```python
from build123d import *

# Parameters (mm, degrees)
BOSS_EXTRUDE1_DEPTH = 17.5
SKETCH2_W           = 20
SKETCH2_H           = 20
CUT_EXTRUDE1_DEPTH  = 64.492125496
SKETCH3_R           = 2
CUT_EXTRUDE2_DEPTH  = 71.356236397
CHAMFER1_SIZE       = 3
CHAMFER2_SIZE       = 5
FILLET1_RADIUS      = 6
FILLET1_LENGTH      = 5
SKETCH4_R           = 2.5
CUT_EXTRUDE3_DEPTH  = 35
FILLET2_R           = 5
FILLET3_R           = 1


with BuildPart() as part:
    # Sketch1 → Boss-Extrude1 (new, symmetric)
    with BuildSketch(Plane(origin=(0, 0, 0), x_dir=(0, 0, -1), z_dir=(1, 0, 0))):
        Polygon((0, 0), (-35, 0), (-35, -20), (-12, -20), (-12, -50), (0, -50), align=None)
    extrude(amount=BOSS_EXTRUDE1_DEPTH, both=True)

    # Sketch2 → Cut-Extrude1 (cut, through all)
    with BuildSketch(Plane(origin=(0, 0, 0), x_dir=(-1, 0, 0), z_dir=(0, 0, -1))):
        Polygon((17.5, -25), (2.5, -30.459553514), (2.5, -50), (17.5, -50), align=None)
        Polygon((-17.5, -50), (-17.5, -25), (-2.5, -30.459553514), (-2.5, -50), align=None)
        with Locations((0, -10)):
            Rectangle(SKETCH2_W, SKETCH2_H)
    extrude(amount=-CUT_EXTRUDE1_DEPTH, mode=Mode.SUBTRACT)

    # Sketch3 → Cut-Extrude2 (cut, through all)
    with BuildSketch(Plane.ZY.offset(17.5)):
        with Locations((5, -8)):
            Circle(SKETCH3_R)
        with Locations((30, -8)):
            Circle(SKETCH3_R)
    extrude(amount=-CUT_EXTRUDE2_DEPTH, mode=Mode.SUBTRACT)

    # Chamfer1
    chamfer1_edges = [part.edges().sort_by_distance(p)[0] for p in [
        (13.75, -20, 12),
        (13.75, -20, 35),
        (13.75, 0, 35),
        (13.75, 0, 0),
        (-13.75, -20, 12),
        (-13.75, -20, 35),
        (-13.75, 0, 35),
        (-13.75, 0, 0),
    ]]
    chamfer(chamfer1_edges, length=CHAMFER1_SIZE)

    # Chamfer2
    chamfer2_edges = [part.edges().sort_by_distance(p)[0] for p in [
        (-10, -20, 6),
        (10, -20, 6),
    ]]
    chamfer(chamfer2_edges, length=CHAMFER2_SIZE)

    # Fillet1: full round fillet: the end face becomes a half cylinder, R = half its width
    fillet1_face = Plane((0, -50, 6), x_dir=(1, 0, 0), z_dir=(0, -1, 0))  # on the end face: x along it, z out of the body
    fillet1_slab = fillet1_face.offset(-FILLET1_RADIUS / 2) * Box(FILLET1_LENGTH, 2 * FILLET1_RADIUS, FILLET1_RADIUS, mode=Mode.PRIVATE)  # the body's end, R deep
    fillet1_round = Plane((0, -44, 6), x_dir=(0, -1, 0), z_dir=(1, 0, 0)) * Cylinder(FILLET1_RADIUS, FILLET1_LENGTH, mode=Mode.PRIVATE)  # its axis R under the face
    add(fillet1_slab - fillet1_round, mode=Mode.SUBTRACT)

    # Sketch4 → Cut-Extrude3 (cut)
    with BuildSketch(Plane(origin=(2.5, 0, 0), x_dir=(0, 0, -1), z_dir=(1, 0, 0))):
        with Locations(Location((-6, -44, 0), (0, 0, 90))):
            Circle(SKETCH4_R)
    extrude(amount=-CUT_EXTRUDE3_DEPTH, mode=Mode.SUBTRACT)

    # Fillet2
    # the kernel refuses this fillet: 5 mm, written as the material it adds along each edge
    with BuildSketch(Plane(origin=(10, -35.5, 12), x_dir=(-1, 0, 0), z_dir=(0, 1, 0))) as fillet2_piece_1_section:
        with BuildLine():
            CenterArc((FILLET2_R, FILLET2_R), FILLET2_R, 180, 90)
            Line((0, FILLET2_R), (0, 0))
            Line((0, 0), (FILLET2_R, 0))
        make_face()
    fillet2_piece_1 = extrude(amount=33, mode=Mode.PRIVATE)
    fillet2_piece_1 = split(fillet2_piece_1, bisect_by=Plane(origin=(9.996559124, -19.16276417, 15.83723583), z_dir=(0, -0.7071067811865476, 0.7071067811865476)), keep=Keep.TOP, mode=Mode.PRIVATE)
    fillet2_piece_1 = split(fillet2_piece_1, bisect_by=Plane(origin=(9.996559124, -20, 16.11631444), z_dir=(0, 1, 0)), keep=Keep.TOP, mode=Mode.PRIVATE)
    add(fillet2_piece_1)
    with BuildSketch(Plane(origin=(10, -35.5, 12), x_dir=(-1, 0, 0), z_dir=(0, 1, 0))) as fillet2_piece_2_section:
        with BuildLine():
            CenterArc((FILLET2_R, FILLET2_R), FILLET2_R, 180, 90)
            Line((0, FILLET2_R), (0, 0))
            Line((0, 0), (FILLET2_R, 0))
        make_face()
    fillet2_piece_2 = extrude(amount=33, mode=Mode.PRIVATE)
    fillet2_piece_2 = split(fillet2_piece_2, bisect_by=Plane(origin=(8.541566655, -21.793394373, 13.206605627), z_dir=(0, 0.7071067811865476, -0.7071067811865476)), keep=Keep.TOP, mode=Mode.PRIVATE)
    fillet2_piece_2 = split(fillet2_piece_2, bisect_by=Plane(origin=(8.541566655, -20, 12.608807503), z_dir=(0, -1, 0)), keep=Keep.TOP, mode=Mode.PRIVATE)
    add(fillet2_piece_2)
    with BuildSketch(Plane(origin=(10, -35.5, 12), x_dir=(-1, 0, 0), z_dir=(0, 1, 0))) as fillet2_piece_3_section:
        with BuildLine():
            CenterArc((FILLET2_R, FILLET2_R), FILLET2_R, 180, 90)
            Line((0, FILLET2_R), (0, 0))
            Line((0, 0), (FILLET2_R, 0))
        make_face()
    fillet2_piece_3 = extrude(amount=33, mode=Mode.PRIVATE)
    fillet2_piece_3 = split(fillet2_piece_3, bisect_by=Plane(origin=(8.131124987, -16.868875013, 13.270711332), z_dir=(0.7071067811865476, -0.7071067811865476, 0)), keep=Keep.TOP, mode=Mode.PRIVATE)
    fillet2_piece_3 = split(fillet2_piece_3, bisect_by=Plane(origin=(9.156989341, -19.812014017, 15.187985983), z_dir=(0, 0.7071067811865476, -0.7071067811865476)), keep=Keep.TOP, mode=Mode.PRIVATE)
    fillet2_piece_3 = split(fillet2_piece_3, bisect_by=Plane(origin=(9.156989341, -20, 13.270711332), z_dir=(0, 1, 0)), keep=Keep.TOP, mode=Mode.PRIVATE)
    add(fillet2_piece_3)
    with BuildSketch(Plane(origin=(-10, -35.5, 12), x_dir=(0, 0, 1), z_dir=(0, 1, 0))) as fillet2_piece_4_section:
        with BuildLine():
            CenterArc((FILLET2_R, FILLET2_R), FILLET2_R, 180, 90)
            Line((0, FILLET2_R), (0, 0))
            Line((0, 0), (FILLET2_R, 0))
        make_face()
    fillet2_piece_4 = extrude(amount=33, mode=Mode.PRIVATE)
    fillet2_piece_4 = split(fillet2_piece_4, bisect_by=Plane(origin=(-8.541566654, -21.793394373, 13.206605627), z_dir=(0, 0.7071067811865476, -0.7071067811865476)), keep=Keep.TOP, mode=Mode.PRIVATE)
    fillet2_piece_4 = split(fillet2_piece_4, bisect_by=Plane(origin=(-8.541566654, -20, 12.608807503), z_dir=(0, -1, 0)), keep=Keep.TOP, mode=Mode.PRIVATE)
    add(fillet2_piece_4)
    with BuildSketch(Plane(origin=(-10, -35.5, 12), x_dir=(0, 0, 1), z_dir=(0, 1, 0))) as fillet2_piece_5_section:
        with BuildLine():
            CenterArc((FILLET2_R, FILLET2_R), FILLET2_R, 180, 90)
            Line((0, FILLET2_R), (0, 0))
            Line((0, 0), (FILLET2_R, 0))
        make_face()
    fillet2_piece_5 = extrude(amount=33, mode=Mode.PRIVATE)
    fillet2_piece_5 = split(fillet2_piece_5, bisect_by=Plane(origin=(-9.996559123, -19.16276417, 15.83723583), z_dir=(0, -0.7071067811865476, 0.7071067811865476)), keep=Keep.TOP, mode=Mode.PRIVATE)
    fillet2_piece_5 = split(fillet2_piece_5, bisect_by=Plane(origin=(-9.996559123, -20, 16.11631444), z_dir=(0, 1, 0)), keep=Keep.TOP, mode=Mode.PRIVATE)
    add(fillet2_piece_5)
    with BuildSketch(Plane(origin=(-10, -35.5, 12), x_dir=(0, 0, 1), z_dir=(0, 1, 0))) as fillet2_piece_6_section:
        with BuildLine():
            CenterArc((FILLET2_R, FILLET2_R), FILLET2_R, 180, 90)
            Line((0, FILLET2_R), (0, 0))
            Line((0, 0), (FILLET2_R, 0))
        make_face()
    fillet2_piece_6 = extrude(amount=33, mode=Mode.PRIVATE)
    fillet2_piece_6 = split(fillet2_piece_6, bisect_by=Plane(origin=(-9.156989342, -19.812014017, 15.187985983), z_dir=(0, 0.7071067811865476, -0.7071067811865476)), keep=Keep.TOP, mode=Mode.PRIVATE)
    fillet2_piece_6 = split(fillet2_piece_6, bisect_by=Plane(origin=(-8.131124988, -16.868875012, 13.270711332), z_dir=(-0.7071067811865476, -0.7071067811865476, 0)), keep=Keep.TOP, mode=Mode.PRIVATE)
    fillet2_piece_6 = split(fillet2_piece_6, bisect_by=Plane(origin=(-9.156989342, -20, 13.270711332), z_dir=(0, 1, 0)), keep=Keep.TOP, mode=Mode.PRIVATE)
    add(fillet2_piece_6)
    with BuildSketch(Plane(origin=(2.5, -30.459553514, 0), x_dir=(0, -1, 0), z_dir=(0, 0, 1)), Plane(origin=(-2.5, -30.459553514, 0), x_dir=(-0.9396926207859091, 0.34202014332566677, 0), z_dir=(0, 0, 1))) as fillet2_piece_7:
        with BuildLine():
            CenterArc((FILLET2_R * 0.70020753821, FILLET2_R), FILLET2_R, 200, 70)
            Line((-FILLET2_R * 0.239485082576, FILLET2_R * 0.657979856674), (0, 0))
            Line((0, 0), (FILLET2_R * 0.70020753821, 0))
        make_face()
    extrude(amount=12)
    # the kernel refuses this fillet: 5 mm, written as the material it takes off along each edge
    with BuildSketch(Plane(origin=(17.5, -25, -8.752594228), x_dir=(0, 1, 0), z_dir=(0, 0, 1))) as fillet2_2_piece_1:
        with BuildLine():
            CenterArc((FILLET2_R * 0.70020753821, FILLET2_R), FILLET2_R, 200, 70)
            Line((-FILLET2_R * 0.239485082576, FILLET2_R * 0.657979856674), (0, 0))
            Line((0, 0), (FILLET2_R * 0.70020753821, 0))
        make_face()
    extrude(amount=29.505188455, mode=Mode.SUBTRACT)
    with BuildSketch(Plane(origin=(-17.5, -25, -8.752594228), x_dir=(0, 1, 0), z_dir=(0, 0, 1))) as fillet2_2_piece_2:
        with BuildLine():
            CenterArc((FILLET2_R * 0.70020753821, -FILLET2_R), FILLET2_R, 90, 70)
            Line((-FILLET2_R * 0.239485082576, -FILLET2_R * 0.657979856674), (0, 0))
            Line((0, 0), (FILLET2_R * 0.70020753821, 0))
        make_face()
    extrude(amount=29.505188455, mode=Mode.SUBTRACT)

    # Fillet3
    fillet3_edges = [part.edges().sort_by_distance(p)[0] for p in [
        (11.134684772, -23, 12),
        (13.541287847, -20, 15),
        (13.75, -20, 32),
        (13.75, -17, 35),
        (13.75, 0, 32),
        (13.75, 0, 3),
        (13.75, -3, 0),
        (13.75, -3, 35),
        (-13.75, -20, 32),
        (-13.541287847, -20, 15),
        (-11.134684772, -23, 12),
        (-13.75, -3, 0),
        (-13.75, 0, 3),
        (-13.75, 0, 32),
        (-13.75, -3, 35),
        (-13.75, -17, 35),
    ]]
    fillet(fillet3_edges, radius=FILLET3_R)


solid = part.part
```
Could you check a few things on this model? Use its own coordinates, in mm. A direction names the side the tool comes from. Round coordinates to 2 decimals unless told otherwise and drop trailing zeros. Loops run counter-clockwise (first coordinate to the right, second up) from the corner with the lowest first, then second, coordinate; pieces in that order, holes last. Notation, with made-up numbers: M -1.5,31 L 8.5,31 A4 cw 8.5,35 Z; hole C -24,-9 d3. An arc over 180 degrees is marked long. Write item = value, one per line.
1. I need wall thicknesses on probe 1 along X at (y, z) = (-13, 28); probe 2 along X at (y, z) = (-37, 5); probe 3 along Y at (x, z) = (15, 30). Which ranges of each line are inside material? Lowest first, please.
Results below:
probe_1 = -17.5 to -10, 10 to 17.5
probe_2 = -2.5 to 2.5
probe_3 = -20 to -10, -6 to 0
2. I want a section at C-C, the plane x = -15. Write out the boundary of the cut face in (y, z).
Results below:
outline = M -25.83,0 L -3.41,0 A1 ccw -2.71,0.29 L -0.29,2.71 A1 ccw 0,3.41 L 0,31.59 A1 ccw -0.29,32.29 L -2.71,34.71 A1 ccw -3.41,35 L -16.59,35 A1 ccw -17.29,34.71 L -19.71,32.29 A1 ccw -20,31.59 L -20,15.41 A1 cw -20.29,14.71 L -22.71,12.29 A1 cw -23.41,12 L -25.83,12 Z; hole C -8,5 d4; hole C -8,30 d4
3. Thinking about a two-plate mould opening in Z: for faces 6 (the face through (13.697, -7.399, 31.908)), 7 (the face through (14, -1, 2)), 8 (the face through (-14, -2, 34)), which applies, +Z half, -Z half, draft (parallel to the pull), parting line (faces both ways), or undercut?
Results below:
face_6 = undercut
face_7 = -Z half
face_8 = +Z half
4. Will these pins go through, and if not, where does the flat tip stop? P1, Ø2.5, axis at x = -14, z = 24, coming from the -Y side; P2, Ø5, axis at x = 0, z = 4.5, coming from the +Y side; P3, Ø13, axis at y = -42, z = 9, coming from the -X side.
Results below:
P1 = -20
P2 = -20
P3 = -2.5
5. Which directions (+Z, -Z, +X, -X, +Y, -Y) give clear straight access to the entire face, cutting with the end or side of a thin tool? Please do faces 1 (the face through (8, -17, 6)), 2 (the face through (14, -20, 23)), 3 (the face through (9, -19, 14)), 4 (the face through (0, -29, 12)), 5 (the face through (2.5, -40, 6)).
Results below:
face_1 = +Z, -Z, +Y
face_2 = +Z, +X, -X, -Y
face_3 = +Z, +Y, -Y
face_4 = +Z, -Y
face_5 = +Z, -Z, +X, -Y
6. I want a section at A-A, the plane z = 30. Write out the boundary of the cut face in (x, y).
Results below:
outline = M -17.5,-20 L -10,-20 L -10,-10 L -17.5,-10 Z; M -17.5,-6 L -10,-6 L -10,0 L -17.5,0 Z; M 10,-20 L 17.5,-20 L 17.5,-10 L 10,-10 Z; M 10,-6 L 17.5,-6 L 17.5,0 L 10,0 Z
7. I want a section at B-B, the plane y = -8. Write out the boundary of the cut face in (x, z).
Results below:
outline = M -17.5,0 L -10,0 L -10,3 L -17.5,3 Z; M -17.5,7 L -10,7 L -10,28 L -17.5,28 Z; M -17.5,32 L -10,32 L -10,35 L -17.5,35 Z; M 10,0 L 17.5,0 L 17.5,3 L 10,3 Z; M 10,7 L 17.5,7 L 17.5,28 L 10,28 Z; M 10,32 L 17.5,32 L 17.5,35 L 10,35 Z
8. I want a section at D-D, the plane y = -43. Write out the boundary of the cut face in (x, z).
Results below:
outline = M -2.5,0 L 2.5,0 L 2.5,3.71 L -2.5,3.71 Z; M -2.5,8.29 L 2.5,8.29 L 2.5,12 L -2.5,12 Z
